```python
from build123d import *

# Parameters (mm, degrees)
F0_W     = 60.007502
F0_H     = 87.23982
F0_R     = 5.379351
F1_DEPTH = 50.8
F3_DEPTH = 40.894
F5_DEPTH = 27.686
F6_D     = 20.32


with BuildPart() as f1:
    # F0 (on Top) → F1 (new body)
    with BuildSketch(Plane.XY):
        with Locations((-0.722982, -9.519262)):
            Rectangle(F0_W, F0_H)
        with Locations((0, -45.909356)):
            Circle(F0_R, mode=Mode.SUBTRACT)
        with Locations((0, 26.147846)):
            Circle(F0_R, mode=Mode.SUBTRACT)
    extrude(amount=F1_DEPTH)

    # F2 (on face) → F3 (join)
    with BuildSketch(Plane(origin=(-30.726733, 0, 0), x_dir=(0, -1, 0), z_dir=(-1, 0, 0))):
        with BuildLine():
            ThreePointArc((28.075797, 50.8), (12.170195, 34.093327), (-3.735408, 50.8))
            Line((-3.735408, 50.8), (-8.281821, 50.8))
            ThreePointArc((-8.281821, 50.8), (12.098354, 27.846321), (32.47853, 50.8))
            Line((32.47853, 50.8), (28.075797, 50.8))
        make_face()
    extrude(amount=F3_DEPTH)

    # F4 (on face) → F5 (join)
    with BuildSketch(Plane.YZ.offset(29.280769)):
        with BuildLine():
            Line((-26.553022, 50.8), (-31.606492, 50.8))
            ThreePointArc((-31.606492, 50.8), (-11.361636, 30.385585), (8.88322, 50.8))
            Line((8.88322, 50.8), (4.536318, 50.8))
            ThreePointArc((4.536318, 50.8), (-11.008352, 35.169395), (-26.553022, 50.8))
        make_face()
    extrude(amount=F5_DEPTH)

    # F6 (through all)
    with Locations(Plane.YZ.offset(29.280769)):
        with Locations((-11.356696, 45.533322)):
            Hole(F6_D / 2)


solid = f1.part
```
The model under review builds one solid part; all positions refer to its coordinate system, in mm. A direction names the side the tool comes from. Round coordinates to 2 decimals unless told otherwise and drop trailing zeros. Write each loop counter-clockwise with the first axis right and the second up, starting at its lowest first coordinate (ties: lowest second). Pieces come first, ordered by that corner, then holes. Notation, with made-up numbers: (60, 82) - (70, 82) arc R21 cw to (70, 89) - close; hole circle Ø9 at (3.25, 52). An arc over 180 degrees is marked (long way). Use one line per item in the form item = value.
Q1. Insertion check: pin 1 Ø15 at (y, z) = (-3, 23) entering from +X; pin 2 Ø8 at (x, y) = (-49.5, -19.5) entering from +Z; pin 3 Ø4 at (y, z) = (-12, 15) entering from -X. Each pin has a flat end and moves straight along its axis. Give the tip position at first contact, or say it passes through.
Answer key:
pin_1 = 29.28
pin_2 = 38.83
pin_3 = -30.73
Q2. Consider section A-A (z = 41). State the section outline as (x, y) points.
Answer key:
outline = (-71.62, -31.25) - (-30.73, -31.25) - (-30.73, -53.14) - (29.28, -53.14) - (29.28, -29.17) - (56.97, -29.17) - (56.97, -23.14) - (29.28, -23.14) - (29.28, -20.45) - (-30.73, -20.45) - (-30.73, -25.3) - (-71.62, -25.3) - close; (-71.62, 0.96) - (-30.73, 0.96) - (-30.73, -2.26) - (29.28, -2.26) - (29.28, 1.13) - (56.97, 1.13) - (56.97, 6.45) - (29.28, 6.45) - (29.28, 34.1) - (-30.73, 34.1) - (-30.73, 7.06) - (-71.62, 7.06) - close; hole circle Ø10.76 at (0, -45.91); hole circle Ø10.76 at (0, 26.15)
Q3. Consider section B-B (x = 0). State the section outline as (y, z) points, and give its area (3 significant figures).
Answer key:
outline = (-53.14, 0) - (-51.29, 0) - (-51.29, 50.8) - (-53.14, 50.8) - close; (-40.53, 0) - (20.77, 0) - (20.77, 50.8) - (-2.67, 50.8) arc R10.16 cw (long way) to (-20.05, 50.8) - (-40.53, 50.8) - close; (31.53, 0) - (34.1, 0) - (34.1, 50.8) - (31.53, 50.8) - close
area = 3,070 mm2
Q4. Tool access review of faces 4 (the flat face through (29.281, -3, 39)), 5 (the flat face through (29.281, -10, 19)), 6 (the flat face through (-30.727, -10, 19)): name each direction out of +Z, -Z, +X, -X, +Y, -Y from which nothing blocks a thin tool from reaching the whole face with its end or side.
Answer key:
face_4 = +Z, +X
face_5 = -Z, +X
face_6 = -Z, -X
Q5. Consider section C-C (y = -48). State the section outline as (x, z) points, and give its area (3 significant figures).
Answer key:
outline = (-30.73, 0) - (-4.96, 0) - (-4.96, 50.8) - (-30.73, 50.8) - close; (4.96, 0) - (29.28, 0) - (29.28, 50.8) - (4.96, 50.8) - close
area = 2,540 mm2
Q6. Consider section D-D (z = 14). State the section outline as (x, y) points, and give its area (3 significant figures).
Answer key:
outline = (-30.73, -53.14) - (29.28, -53.14) - (29.28, 34.1) - (-30.73, 34.1) - close; hole circle Ø10.76 at (0, -45.91); hole circle Ø10.76 at (0, 26.15)
area = 5,050 mm2
Q7. For line 1 (Y direction, x = 0, z = 14); line 2 (X direction, y = 26, z = 31); line 3 (X direction, y = -46.5, z = 43.5), list the stretches that pass through material, from the lowest coordinate up. Write a range as [from, to].
Answer key:
line_1 = [-53.14, -51.29], [-40.53, 20.77], [31.53, 34.1]
line_2 = [-30.73, -5.38], [5.38, 29.28]
line_3 = [-30.73, -5.35], [5.35, 29.28]
Q8. Draft analysis for pull direction Z (two halves, no side actions). For faces 1 (the cylindrical face through (-1.143, -11.056, 35.378)), 2 (the flat face through (-1, 34.101, 25)), 3 (the flat face through (-1, -9, 0)), state which applies: +Z half, -Z half, draft (parallel to the pull), parting line (faces both ways), or undercut.
Answer key:
face_1 = undercut
face_2 = draft
face_3 = -Z half
